The model under review builds one solid part; all positions refer to its coordinate system, in mm. A direction names the side the tool comes from. Round coordinates to 2 decimals unless told otherwise and drop trailing zeros. Order: outer loops, then holes, each group sorted by start corner. A loop starts at its lowest first (then second) coordinate and runs counter-clockwise, first axis right, second up.
```python
from build123d import *

# Parameters (mm, degrees)
BOSS_EXTRUDE1_DEPTH = 164
BOSS_EXTRUDE2_DEPTH = 1.6


with BuildPart() as part:
    # Sketch1 → Boss-Extrude1 (new body)
    with BuildSketch(Plane.XY):
        Polygon((-27, 10), (-27, 0), (27, 0), (27, 10), (0.8, 10), (0.8, 7), (-0.8, 7), (-0.8, 10), align=None)
    extrude(amount=BOSS_EXTRUDE1_DEPTH)

    # Sketch2 → Boss-Extrude2 (add)
    with BuildSketch(Plane(origin=(27, 0, 0), x_dir=(0, 0, -1), z_dir=(1, 0, 0))):
        Polygon((-151, 0), (-150.85, 5.5), (-146.55, 5.5), (-146.4, 0), align=None)
        Polygon((-13.15, 5.5), (-17.45, 5.5), (-17.6, 0), (-13, 0), align=None)
        Polygon((-84.3, 0), (-84.15, 5.5), (-79.85, 5.5), (-79.7, 0), align=None)
    boss_extrude2 = extrude(amount=BOSS_EXTRUDE2_DEPTH)

    # Mirror1: Boss-Extrude2 across plane
    add(boss_extrude2.mirror(Plane(origin=(0, 0, 0), x_dir=(0, 0, 1), z_dir=(1, 0, 0))))


solid = part.part
```
(1) To check wall thickness, follow probe 1 along X at (y, z) = (8.5, 57.5); probe 2 along X at (y, z) = (1, 121). State the ranges of each line that lie inside material, in increasing order.
Data:
probe 1: x = -27 to -0.8, 0.8 to 27
probe 2: x = -27 to 27
(2) Draft analysis for pull direction Z (two halves, no side actions). For faces 3 (the flat face through (27, 6, 81)), 4 (the flat face through (0, 5, 164)), 5 (the flat face through (-28.6, 3, 82)), state which applies: pulls with the +Z half, pulls with the -Z half, needs draft (parallel to the pull), parting line crosses it, or undercut.
Data:
face 3: undercut
face 4: pulls with the +Z half
face 5: needs draft
(3) Consider section B-B (y = 3.5). Write out the cut boundary in (x, z).
Data:
outline: (-28.6, 13.1) - (-27, 13.1) - (-27, 0) - (27, 0) - (27, 13.1) - (28.6, 13.1) - (28.6, 17.5) - (27, 17.5) - (27, 79.8) - (28.6, 79.8) - (28.6, 84.2) - (27, 84.2) - (27, 146.5) - (28.6, 146.5) - (28.6, 150.9) - (27, 150.9) - (27, 164) - (-27, 164) - (-27, 150.9) - (-28.6, 150.9) - (-28.6, 146.5) - (-27, 146.5) - (-27, 84.2) - (-28.6, 84.2) - (-28.6, 79.8) - (-27, 79.8) - (-27, 17.5) - (-28.6, 17.5) - close
(4) Consider section C-C (z = 43.5). Write out the cut boundary in (x, y).
Data:
outline: (-27, 0) - (27, 0) - (27, 10) - (0.8, 10) - (0.8, 7) - (-0.8, 7) - (-0.8, 10) - (-27, 10) - close
(5) Insertion check: pin 1 (0.5 mm diameter, centred on x = 0, z = 65.5, fed in from +Y); pin 2 (1.3 mm diameter, centred on x = -28, z = 149.5, fed in from +Y); pin 3 (1.5 mm diameter, centred on y = 8.5, z = 92, fed in from +X). Each pin has a flat end and moves straight along its axis. Give the tip position at first contact, or say it passes through.
Data:
pin 1: stops at y = 7
pin 2: stops at y = 5.5
pin 3: stops at x = 27
(6) For faces 1 (the flat face through (0.8, 9, 81)), 2 (the flat face through (28.6, 3, 15)), list the 3-axis set-ups (+Z, -Z, +X, -X, +Y, -Y) from which the entire face can be reached by the end or side of a thin tool; tool diameter is ignored.
Data:
face 1: +Z, -Z, +Y
face 2: +Z, -Z, +X, +Y, -Y
(7) Consider section A-A (z = 82). Write out the cut boundary in (x, y), and give its area (3 significant figures).
Data:
outline: (-28.6, 0) - (28.6, 0) - (28.6, 5.5) - (27, 5.5) - (27, 10) - (0.8, 10) - (0.8, 7) - (-0.8, 7) - (-0.8, 10) - (-27, 10) - (-27, 5.5) - (-28.6, 5.5) - close
area: 553 mm2
